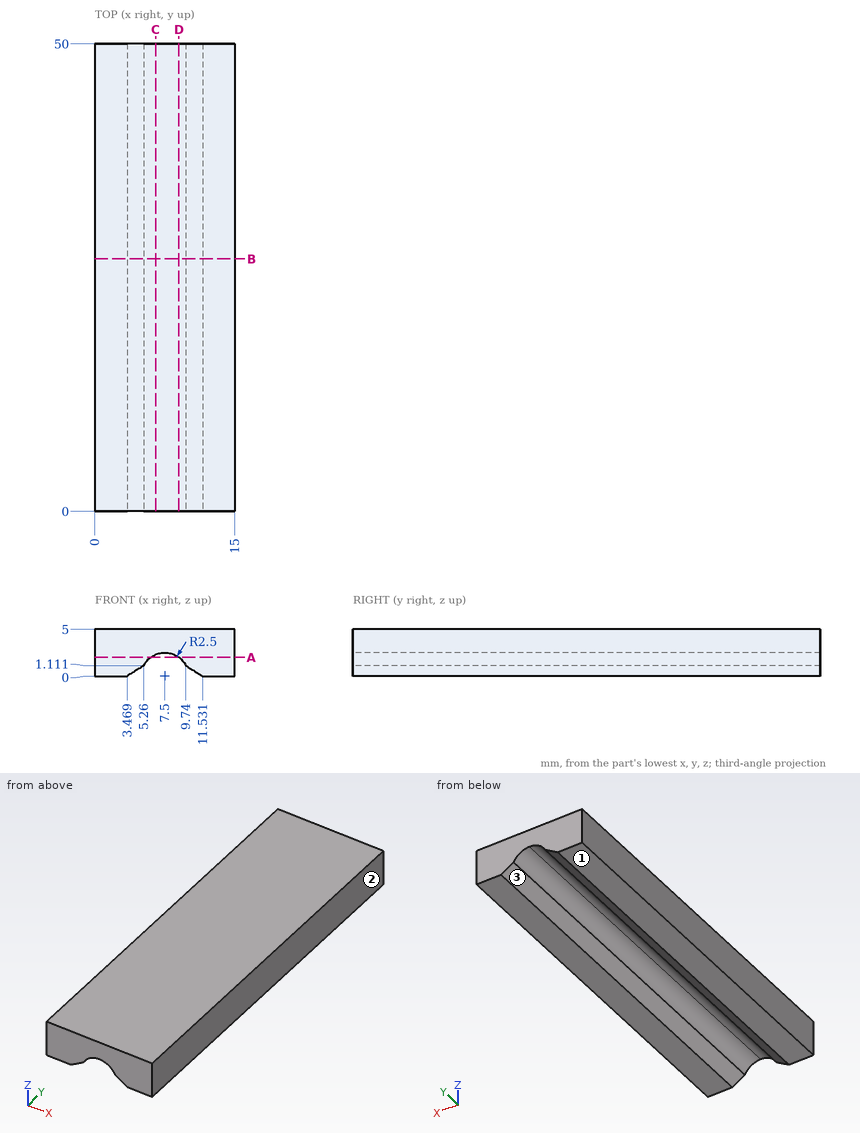
Could you check a few things on this drawing? It's one solid part, dimensions in mm from its lowest x, y, z. Coordinates: 2 decimals unless noted, no trailing zeros. Write each loop counter-clockwise with the first axis right and the second up, starting at its lowest first coordinate (ties: lowest second). Pieces come first, ordered by that corner, then holes.
1) If we section it at A-A (z = 2): List the corners of the cut face in (x, y) for me, plus the area to 3 significant figures.
Filled in:
outline: (0, 0) - (6, 0) - (6, 50) - (0, 50) - close; (9, 0) - (15, 0) - (15, 50) - (9, 50) - close
area: 600 mm2
2) If I drill on line 1 (X direction, y = 46, z = 2.1) (1 decimal); line 2 (X direction, y = 13, z = 2); line 3 (Z direction, x = 8.5, y = 12), over which ranges is the centre line in solid material (lowest first)?
Filled in:
line 1: x = 0 to 6.1, 8.9 to 15
line 2: x = 0 to 6, 9 to 15
line 3: z = 2.29 to 5
3) Thinking about a two-plate mould opening in X: for the marked faces 1, 2 and 3, which applies, +X half, -X half, draft (parallel to the pull), parting line (faces both ways), or undercut?
Filled in:
face 1: draft
face 2: +X half
face 3: undercut
4) If we section it at B-B (y = 27): List the corners of the cut face in (x, z) for me.
Filled in:
outline: (0, 0) - (3.47, 0) - (5.26, 1.11) arc R2.5 cw to (9.74, 1.11) - (11.53, 0) - (15, 0) - (15, 5) - (0, 5) - close
5) If we section it at C-C (x = 6.5): List the corners of the cut face in (y, z) for me.
Filled in:
outline: (0, 2.29) - (50, 2.29) - (50, 5) - (0, 5) - close
6) If we section it at D-D (x = 9): List the corners of the cut face in (y, z) for me.
Filled in:
outline: (0, 2) - (50, 2) - (50, 5) - (0, 5) - close
7) I'm going to push a flat-ended pin straight in: pin 1 (1.5 mm diameter, centred on y = 32.5, z = 3, fed in from -X). Where does the tip first touch, or does it pass through?
Filled in:
pin 1: stops at x = 0
